Study the drawing (mm; zero at the part's minimum x, y, z) and answer. A direction names the side the tool comes from. Round coordinates to 2 decimals unless told otherwise and drop trailing zeros. Write each loop counter-clockwise with the first axis right and the second up, starting at its lowest first coordinate (ties: lowest second). Pieces come first, ordered by that corner, then holes. Notation, with made-up numbers: M 84,-20.75 L 138,-20.75 A28 ccw 138,11.25 Z; hole C 40.5,16.5 d5. An arc over 180 degrees is marked long. Write each question's results on one line, items separated by ' | '.
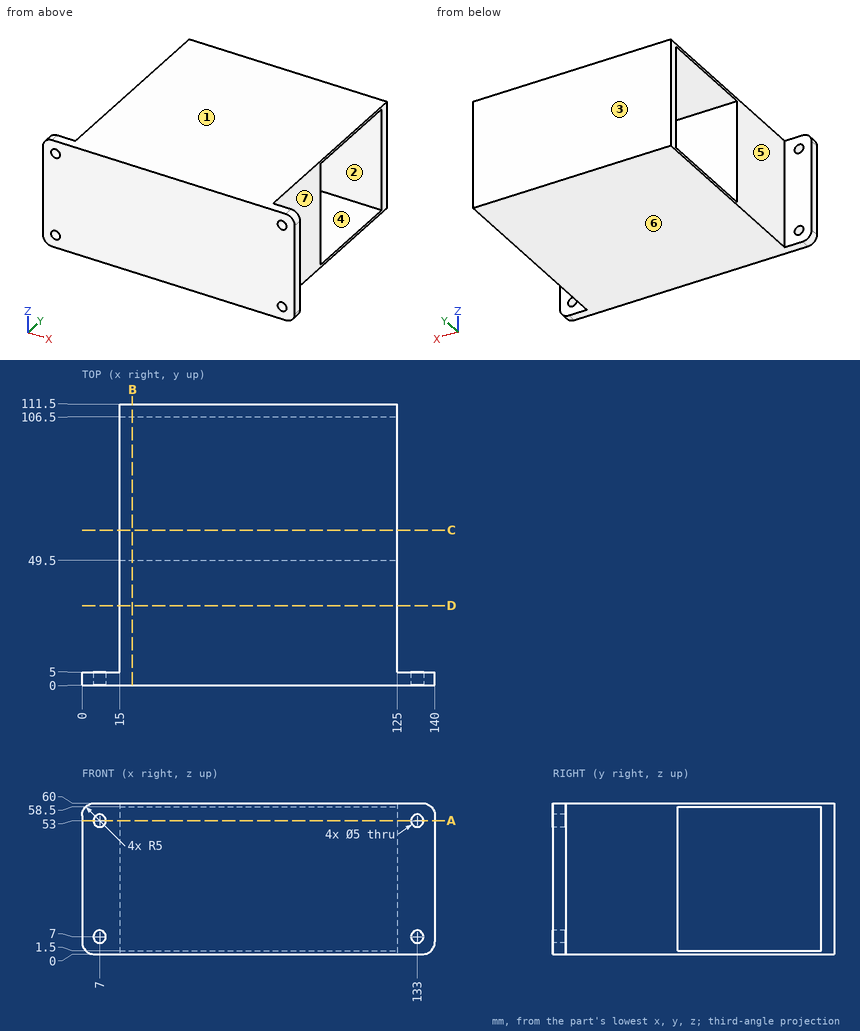
1) Section A-A (z = 53) is taken. Determine the outline of the cut face in (x, y).
Return value:
outline: M 0,0 L 4.5,0 L 4.5,5 L 0,5 Z; M 9.5,0 L 130.5,0 L 130.5,5 L 125,5 L 125,49.5 L 15,49.5 L 15,5 L 9.5,5 Z; M 15,106.5 L 125,106.5 L 125,111.5 L 15,111.5 Z; M 135.5,0 L 140,0 L 140,5 L 135.5,5 Z
2) Each of these flat-tipped pins is pushed along its axis until it touches: pin 1 (4.5 mm diameter, centred on x = 10.5, z = 19.5, fed in from +Y); pin 2 (12 mm diameter, centred on y = 13, z = 10, fed in from -X); pin 3 (3 mm diameter, centred on y = 36, z = 44.5, fed in from +X). Where does it stop, or does it pass through?
Return value:
pin 1: y = 5 | pin 2: x = 15 | pin 3: x = 125
3) Section B-B (x = 20) is taken. Determine the outline of the cut face in (y, z).
Return value:
outline: M 0,0 L 111.5,0 L 111.5,60 L 0,60 Z; hole M 49.5,1.5 L 106.5,1.5 L 106.5,58.5 L 49.5,58.5 Z
4) A tool of negligible diameter and unlimited length cuts with its end or side. For the marked faces 4, 5, 6 and 7, from which of +Z, -Z, +X, -X, +Y, -Y can it reach the whole face along a straight path? Write none if from no direction.
Return value:
face 4: +X, -X | face 5: +Z, -Z, -X, +Y | face 6: -Z, +X, -X, +Y, -Y | face 7: +Z, -Z, +X, +Y
5) Section C-C (y = 61.5) is taken. Determine the outline of the cut face in (x, z).
Return value:
outline: M 15,0 L 125,0 L 125,1.5 L 15,1.5 Z; M 15,58.5 L 125,58.5 L 125,60 L 15,60 Z
6) Section D-D (y = 31.5) is taken. Determine the outline of the cut face in (x, z), then the cut area to 3 significant figures.
Return value:
outline: M 15,0 L 125,0 L 125,60 L 15,60 Z | area: 6,600 mm²
7) Find the intervals of material crossed by line 1 (X direction, y = 3.5, z = 7); line 2 (Z direction, x = 7, y = 1.35); line 3 (Y direction, x = 108.5, z = 29.5), in increasing order.
Return value:
line 1: 0 to 4.5, 9.5 to 130.5, 135.5 to 140 | line 2: 0 to 4.5, 9.5 to 50.5, 55.5 to 60 | line 3: 0 to 49.5, 106.5 to 111.5
8) The mould has two halves that part along Z. Classify the marked faces 1, 2 and 3: +Z half, -Z half, draft (parallel to the pull), parting line (faces both ways), or undercut.
Return value:
face 1: +Z half | face 2: undercut | face 3: draft
